Part print with two shaded views. Sizes in mm from the minimum x, y, z corner. A direction names the side the tool comes from. Round coordinates to 2 decimals unless told otherwise and drop trailing zeros. Order: outer loops, then holes, each group sorted by start corner. A loop starts at its lowest first (then second) coordinate and runs counter-clockwise, first axis right, second up. Notation, with made-up numbers: M 72.25,-30.75 L 91.25,-30.75 A25 ccw 91.25,-13.75 Z; hole C 31,19.25 d5. An arc over 180 degrees is marked long. Return JSON: item names as keys, results as strings. Group by question number.
Item 1: Slice it at A-A on x = 18.27. Write the cut outline in (y, z).
Item 2: Probe line 1 along Z through (x, y) = (64.23, 12.25); line 2 along Z through (x, y) = (18.27, 14); line 3 along X through (y, z) = (1.75, 24). List the from-to ranges inside material, lowest first.
Item 3: Slice it at C-C on y = 15. Give the number of separate pieces and of enclosed holes in the cut face, then the cut area to 3 significant figures.
Item 4: Slice it at D-D on x = 35. Write the cut outline in (y, z), then the cut area to 3 significant figures.
Item 5: Pull direction X, two halves, no side cores. Call the marked faces 4, 5, 6 and 7: pulls with the +X half, pulls with the -X half, needs draft (parallel to the pull), parting line crosses it, or undercut.
Item 6: Which spindle directions (+Z, -Z, +X, -X, +Y, -Y) get a long thin tool onto all of the face, cutting with end or side? Do the marked faces 1, 2 and 3. Say none if no direction does.
Item 7: Slice it at B-B on z = 21. Write the cut outline in (x, y), then the cut area to 3 significant figures.
Item 8: Pin check, flat tips, straight feed: pin 1 Ø5 at (x, z) = (18.27, 4.27) entering from +Y; pin 2 Ø5 at (y, z) = (5, 19.5) entering from -X; pin 3 Ø6 at (y, z) = (4, 15) entering from +X; pin 4 Ø8 at (x, z) = (67.5, 28.5) entering from -Y. Stop position of each tip, or through.
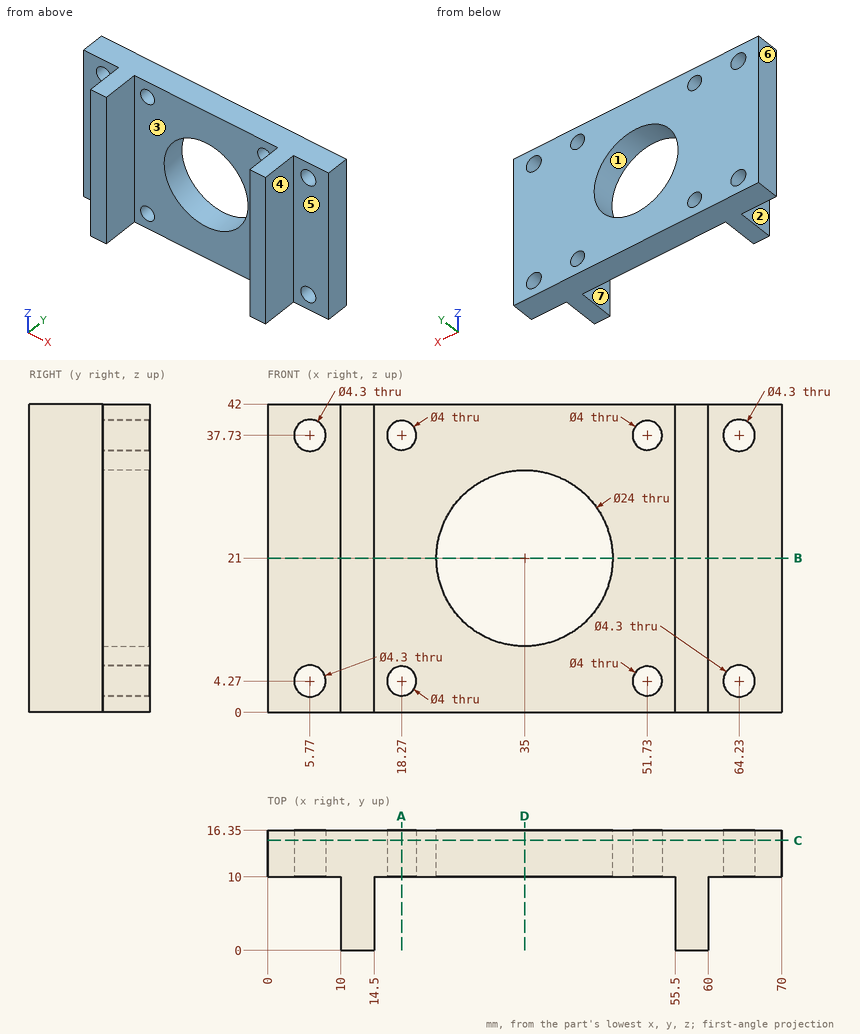
Output values:
{
 "1": {"outline": "M 10,0 L 16.35,0 L 16.35,2.27 L 10,2.27 Z; M 10,6.27 L 16.35,6.27 L 16.35,35.73 L 10,35.73 Z; M 10,39.73 L 16.35,39.73 L 16.35,42 L 10,42 Z"},
 "2": {"line 1": "0 to 2.12, 6.42 to 35.58, 39.88 to 42", "line 2": "0 to 2.27, 6.27 to 35.73, 39.73 to 42", "line 3": "10 to 14.5, 55.5 to 60"},
 "3": {"separate pieces": "1", "enclosed holes": "9", "area": "2,380 mm²"},
 "4": {"outline": "M 10,0 L 16.35,0 L 16.35,9 L 10,9 Z; M 10,33 L 16.35,33 L 16.35,42 L 10,42 Z", "area": "114 mm²"},
 "5": {"face 4": "pulls with the +X half", "face 5": "needs draft", "face 6": "pulls with the -X half", "face 7": "undercut"},
 "6": {"face 1": "+Y, -Y", "face 2": "+Z, -Z, -X, -Y", "face 3": "+Z, -Z, -Y"},
 "7": {"outline": "M 0,10 L 10,10 L 10,0 L 14.5,0 L 14.5,10 L 23,10 L 23,16.35 L 0,16.35 Z; M 47,10 L 55.5,10 L 55.5,0 L 60,0 L 60,10 L 70,10 L 70,16.35 L 47,16.35 Z", "area": "382 mm²"},
 "8": {"pin 1": "y = 16.35", "pin 2": "x = 10", "pin 3": "x = 60", "pin 4": "y = 10"}
}
